Part model, mm, in its own coordinate system. A direction names the side the tool comes from. Round coordinates to 2 decimals unless told otherwise and drop trailing zeros. Loops run counter-clockwise (first coordinate to the right, second up) from the corner with the lowest first, then second, coordinate; pieces in that order, holes last.
(1) Probe probe 1 along X at (y, z) = (-12, 2.25); probe 2 along Y at (x, z) = (23, 4.25); probe 3 along Z at (x, y) = (7.5, -13.25). List the from-to ranges inside material, lowest first.
(2) Flat gauge pins, fed straight in: pin 1 (1.5 mm diameter, centred on x = 16.5, y = -5, fed in from +Z); pin 2 (2 mm diameter, centred on x = 18, y = -4, fed in from -Z); pin 3 (6 mm diameter, centred on x = 25, y = -11.5, fed in from +Z). Where does each tip first touch, or does it go through?
(3) Cut at C-C on y = -7.5. List the corners of the cut face in (x, z), then the cut area to 3 significant figures.
(4) Tool access for faces 4 (the face through (5, -7, 1)), 5 (the face through (21.863, -8, 7)), 6 (the face through (2, -7, 0)): list every direction of +Z, -Z, +X, -X, +Y, -Y with a clear straight run to the whole face (end or side of a thin tool).
(5) Cut at B-B on x = 24. List the corners of the cut face in (y, z).
(6) Mould opens along X. For faces 1 (the face through (30, -1, 4)), 2 (the face through (12, -7, 2.5)), 3 (the face through (11, -15, 10)) say: +X half, -X half, draft (parallel to the pull), parting line (faces both ways), or undercut.
(7) Cut at D-D on z = 10. List the corners of the cut face in (x, y).
(8) Cut at A-A on z = 1.75. List the corners of the cut face in (x, y), then the cut area to 3 significant figures.
from build123d import *

# Parameters (mm, degrees)
F1_DEPTH = 15
F2_W     = 8.1373347121
F2_H     = 10
F3_DEPTH = 25


with BuildPart() as f1:
    # F0 (on Front) → F1 (new body)
    with BuildSketch(Plane.XZ):
        Polygon((0, 20), (0, 0), (5, 0), (5, 2.5), (20, 2.5), (20, 0), (30, 0), (30, 7.5), (12.5, 20), align=None)
    extrude(amount=F1_DEPTH)

    # F2 (on Top) → F3 (cut)
    with BuildSketch(Plane.XY):
        with Locations((25.931332644, -7.5)):
            Rectangle(F2_W, F2_H)
    extrude(amount=F3_DEPTH, mode=Mode.SUBTRACT)


solid = f1.part
Final values:
1. probe 1: x = 0 to 5, 20 to 21.86
1. probe 2: y = -15 to -12.5, -2.5 to 0
1. probe 3: z = 2.5 to 20
2. pin 1: stops at z = 17.68
2. pin 2: stops at z = 2.5
2. pin 3: stops at z = 13.09
3. outline: (0, 0) - (5, 0) - (5, 2.5) - (20, 2.5) - (20, 0) - (21.86, 0) - (21.86, 13.31) - (12.5, 20) - (0, 20) - close
3. area: 368 mm2
4. face 4: -Z, +Y, -Y
4. face 5: +Z, -Z, +X
4. face 6: -Z, +X, -X, +Y, -Y
5. outline: (-15, 0) - (-12.5, 0) - (-12.5, 11.79) - (-15, 11.79) - close; (-2.5, 0) - (0, 0) - (0, 11.79) - (-2.5, 11.79) - close
6. face 1: +X half
6. face 2: undercut
6. face 3: draft
7. outline: (0, -15) - (26.5, -15) - (26.5, -12.5) - (21.86, -12.5) - (21.86, -2.5) - (26.5, -2.5) - (26.5, 0) - (0, 0) - close
8. outline: (0, -15) - (5, -15) - (5, 0) - (0, 0) - close; (20, -15) - (30, -15) - (30, -12.5) - (21.86, -12.5) - (21.86, -2.5) - (30, -2.5) - (30, 0) - (20, 0) - close
8. area: 144 mm2
